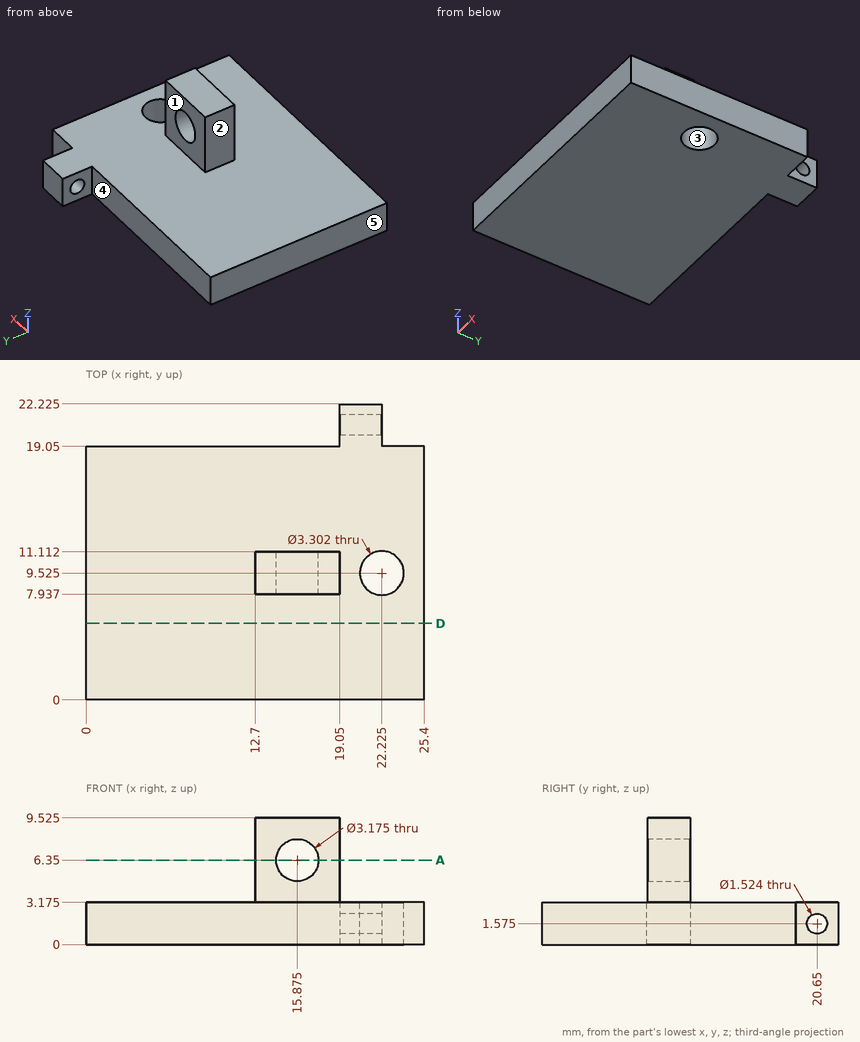
Study the drawing (mm; zero at the part's minimum x, y, z) and answer. A direction names the side the tool comes from. Round coordinates to 2 decimals unless told otherwise and drop trailing zeros. Order: outer loops, then holes, each group sorted by start corner. A loop starts at its lowest first (then second) coordinate and runs counter-clockwise, first axis right, second up. Notation, with made-up numbers: M 65.25,45 L 69.25,45 A15 cw 69.25,66 Z; hole C 85,-35.75 d10. An arc over 180 degrees is marked long. One line per item, written item: value.
Q1. Determine the mould class of the marked faces 1, 2 and 3 for opening direction X: released by +X, released by -X, zero draft, split by the parting line, or undercut.
Derived:
face 1: zero draft
face 2: released by -X
face 3: undercut
Q2. Flat-ended cylindrical pins translate along their axes: pin 1 (2.5 mm diameter, centred on x = 5, z = 2, fed in from +Y); pin 2 (1 mm diameter, centred on y = 20, z = 2, fed in from +X) (1 decimal); pin 3 (3 mm diameter, centred on x = 17, z = 6, fed in from -Y). Find the tip coordinate at first contact, or state that the pin passes through.
Derived:
pin 1: y = 19.05
pin 2: x = 22.2
pin 3: y = 7.94
Q3. Find section D-D on y = 5.75. Write down the section's boundary in (x, z) (1 decimal).
Derived:
outline: M 0,0 L 25.4,0 L 25.4,3.2 L 0,3.2 Z
Q4. Straight lines are drawn through the part: line 1 (X direction, y = 9.7, z = 6.35); line 2 (X direction, y = 9.5, z = 2.75) (1 decimal); line 3 (Z direction, x = 2.25, y = 1) (1 decimal). For each, find the intervals that lie inside material, in ascending order.
Derived:
line 1: 12.7 to 14.29, 17.46 to 19.05
line 2: 0 to 20.6, 23.9 to 25.4
line 3: 0 to 3.2
Q5. For the marked faces 4 and 5, determine the directions among +Z, -Z, +X, -X, +Y, -Y from which every point of the face is accessible in a straight line to the end or side of a thin tool.
Derived:
face 4: +Z, -Z, -X, +Y
face 5: +Z, -Z, -X, +Y, -Y
Q6. Find section A-A on z = 6.35. Write down the section's boundary in (x, y), then the cut area to 3 significant figures.
Derived:
outline: M 12.7,7.94 L 14.29,7.94 L 14.29,11.11 L 12.7,11.11 Z; M 17.46,7.94 L 19.05,7.94 L 19.05,11.11 L 17.46,11.11 Z
area: 10.1 mm²
